from build123d import *

# Parameters (mm, degrees)
SKETCH1_R           = 3.175
BOSS_EXTRUDE1_DEPTH = 3.175


with BuildPart() as part:
    # Sketch1 → Boss-Extrude1 (new body)
    with BuildSketch(Plane(origin=(0, 3.175, 0), x_dir=(1, 0, 0), z_dir=(0, 1, 0))):
        with BuildLine():
            Line((67.238500214, -4.780193669), (67.238500214, 4.780193669))
            ThreePointArc((67.238500214, 4.780193669), (66.859153267, 6.115550693), (65.834422746, 7.052038734))
            Line((65.834422746, 7.052038734), (42.374810083, 18.781845065))
            ThreePointArc((42.374810083, 18.781845065), (41.822459969, 18.982052433), (41.238887551, 19.05))
            Line((41.238887551, 19.05), (-8.361887124, 19.05))
            ThreePointArc((-8.361887124, 19.05), (-8.945459542, 18.982052433), (-9.497809656, 18.781845065))
            Line((-9.497809656, 18.781845065), (-32.957422319, 7.052038734))
            ThreePointArc((-32.957422319, 7.052038734), (-33.98215284, 6.115550693), (-34.361499786, 4.780193669))
            Line((-34.361499786, 4.780193669), (-34.361499786, -4.780193669))
            ThreePointArc((-34.361499786, -4.780193669), (-33.98215284, -6.115550693), (-32.957422319, -7.052038734))
            Line((-32.957422319, -7.052038734), (-9.497809656, -18.781845065))
            ThreePointArc((-9.497809656, -18.781845065), (-8.945459542, -18.982052433), (-8.361887124, -19.05))
            Line((-8.361887124, -19.05), (41.238887551, -19.05))
            ThreePointArc((41.238887551, -19.05), (41.822459969, -18.982052433), (42.374810083, -18.781845065))
            Line((42.374810083, -18.781845065), (65.834422746, -7.052038734))
            ThreePointArc((65.834422746, -7.052038734), (66.859153267, -6.115550693), (67.238500214, -4.780193669))
        make_face()
        with Locations((-28.011499786, 0)):
            Circle(SKETCH1_R, mode=Mode.SUBTRACT)
        with Locations((60.888500214, 0)):
            Circle(SKETCH1_R, mode=Mode.SUBTRACT)
    extrude(amount=-BOSS_EXTRUDE1_DEPTH)


solid = part.part
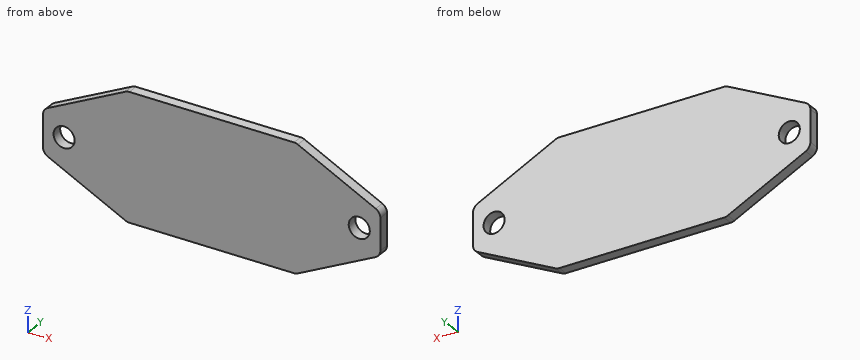
Part model, mm, in its own coordinate system. Round coordinates to 2 decimals unless told otherwise and drop trailing zeros. Write each loop counter-clockwise with the first axis right and the second up, starting at its lowest first coordinate (ties: lowest second). Pieces come first, ordered by that corner, then holes. Notation, with made-up numbers: (3.25, 73.5) - (46.25, 73.5) arc R19 cw to (46.25, 110.5) - close; hole circle Ø1 at (4.5, 42). An arc over 180 degrees is marked (long way). Use CSV: the item, a comma, the result in double quotes.
Item 1: Slice it at B-B, the plane y = 1.5. Count the separate pieces of the cut face and the enclosed holes in it, then the cut area to 3 significant figures.
Results list:
separate pieces,"1"
enclosed holes,"2"
area,"3,160 mm²"
Item 2: Slice it at C-C, the plane z = -8. Write the cut outline in (x, y) (1 decimal), then the cut area to 3 significant figures.
Results list:
outline,"(-31.1, 0) - (63.9, 0) - (63.9, 3.2) - (-31.1, 3.2) - close"
area,"302 mm²"
Item 3: Wall check: L1, parallel to X at y = 1.8, z = 0; L2, parallel to X at y = 2.4, z = 2.5; L3, parallel to X at y = 1.2, z = -5. Give the ranges that are in metal, low to high.
Results list:
L1,"x = -34.36 to -31.19, -24.84 to 57.71, 64.06 to 67.24"
L2,"x = -34.36 to -29.97, -26.05 to 58.93, 62.85 to 67.24"
L3,"x = -34.35 to 67.23"
Item 4: Flat gauge pins, fed straight in: P1, Ø1.5, axis at y = 2.5, z = 8, coming from the +X side; P2, Ø1.5, axis at y = 1, z = -13.5, coming from the -X side. Where does each tip first touch, or does it go through?
Results list:
P1,"stops at x = 65.44"
P2,"stops at x = -21.56"
Item 5: Slice it at A-A, the plane z = 0. Write the cut outline in (x, y) (1 decimal).
Results list:
outline,"(-34.4, 0) - (-31.2, 0) - (-31.2, 3.2) - (-34.4, 3.2) - close; (-24.8, 0) - (57.7, 0) - (57.7, 3.2) - (-24.8, 3.2) - close; (64.1, 0) - (67.2, 0) - (67.2, 3.2) - (64.1, 3.2) - close"
